Here's how the part is built. I have some questions about the finished solid (model axes, mm). Face numbers are marked on the shaded views. Round coordinates to 2 decimals unless told otherwise and drop trailing zeros. Order: outer loops, then holes, each group sorted by start corner. A loop starts at its lowest first (then second) coordinate and runs counter-clockwise, first axis right, second up.
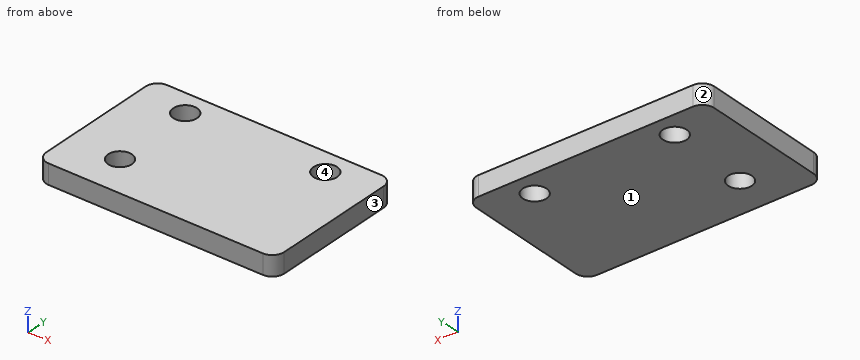
```python
from build123d import *

# Parameters (mm, degrees)
EXTRUDE_1_DEPTH     = 5
SKETCH_2_R          = 3
CUT_EXTRUDE_1_DEPTH = 10
SKETCH_4_R          = 3
CUT_EXTRUDE_2_DEPTH = 10


with BuildPart() as part:
    # 草图1 → 凸台-拉伸1 (new body)
    with BuildSketch(Plane.XY):
        with BuildLine():
            Line((-15.5, 27.5), (38.5, 27.5))
            ThreePointArc((38.5, 27.5), (40.621320344, 26.621320344), (41.5, 24.5))
            Line((41.5, 24.5), (41.5, -7))
            ThreePointArc((41.5, -7), (40.621320344, -9.121320344), (38.5, -10))
            Line((38.5, -10), (33.3, -10))
            Line((33.3, -10), (31.175, -10))
            Line((31.175, -10), (-8.825, -10))
            Line((-8.825, -10), (-15.5, -10))
            ThreePointArc((-15.5, -10), (-17.621320344, -9.121320344), (-18.5, -7))
            Line((-18.5, -7), (-18.5, 24.5))
            ThreePointArc((-18.5, 24.5), (-17.621320344, 26.621320344), (-15.5, 27.5))
        make_face()
    extrude(amount=EXTRUDE_1_DEPTH)

    # 草图2 → 切除-拉伸1 (cut)
    with BuildSketch(Plane.XY.offset(5)):
        with Locations((-6.17, 21.5)):
            Circle(SKETCH_2_R)
        with Locations((29.17, 21.5)):
            Circle(SKETCH_2_R)
    extrude(amount=-CUT_EXTRUDE_1_DEPTH, mode=Mode.SUBTRACT)

    # 草图4 → 切除-拉伸2 (cut)
    with BuildSketch(Plane.XY.offset(5)):
        with Locations((-5.5, 0)):
            Circle(SKETCH_4_R)
    extrude(amount=-CUT_EXTRUDE_2_DEPTH, mode=Mode.SUBTRACT)


solid = part.part
```
1) If we section it at C-C (z = 1.95): Write out the boundary of the cut face in (x, y), plus the area to 3 significant figures.
2) If we section it at B-B (x = 29.17): Write out the boundary of the cut face in (y, z), plus the area to 4 significant figures.
3) If we section it at A-A (y = 21.5): Write out the boundary of the cut face in (x, z).
4) We'd pull the mould along X, two halves only. Please class the marked faces 1, 2, 3 and 4: +X half, -X half, draft (parallel to the pull), parting line (faces both ways), or undercut.
5) I'm going to push a flat-ended pin straight in: pin 1 (5 mm diameter, centred on x = 29.17, y = 21.5, fed in from -Z). Where does the tip first touch, or does it pass through?
6) If we section it at D-D (y = -2): Write out the boundary of the cut face in (x, z).
7) I need wall thicknesses on line 1 (Y direction, x = -5, z = 3.8); line 2 (X direction, y = 19, z = 2.95); line 3 (X direction, y = -0.5, z = 1.95). Which ranges of each line are inside material? Lowest first, please.
Solutions:
1. outline: (-18.5, -7) arc R3 ccw to (-15.5, -10) - (38.5, -10) arc R3 ccw to (41.5, -7) - (41.5, 24.5) arc R3 ccw to (38.5, 27.5) - (-15.5, 27.5) arc R3 ccw to (-18.5, 24.5) - close; hole circle Ø6 at (-6.17, 21.5); hole circle Ø6 at (-5.5, 0); hole circle Ø6 at (29.17, 21.5)
1. area: 2,160 mm2
2. outline: (-10, 0) - (18.5, 0) - (18.5, 5) - (-10, 5) - close; (24.5, 0) - (27.5, 0) - (27.5, 5) - (24.5, 5) - close
2. area: 157.5 mm2
3. outline: (-18.5, 0) - (-9.17, 0) - (-9.17, 5) - (-18.5, 5) - close; (-3.17, 0) - (26.17, 0) - (26.17, 5) - (-3.17, 5) - close; (32.17, 0) - (41.5, 0) - (41.5, 5) - (32.17, 5) - close
4. face 1: draft
4. face 2: -X half
4. face 3: +X half
4. face 4: undercut
5. pin 1: passes through
6. outline: (-18.5, 0) - (-7.74, 0) - (-7.74, 5) - (-18.5, 5) - close; (-3.26, 0) - (41.5, 0) - (41.5, 5) - (-3.26, 5) - close
7. line 1: y = -10 to -2.96, 2.96 to 18.74, 24.26 to 27.5
7. line 2: x = -18.5 to -7.83, -4.51 to 27.51, 30.83 to 41.5
7. line 3: x = -18.5 to -8.46, -2.54 to 41.5
